```python
from build123d import *

# Parameters (mm, degrees)
SKETCH1_R           = 1.6
BOSS_EXTRUDE1_DEPTH = 5
SKETCH2_R           = 2.5
CUT_EXTRUDE1_DEPTH  = 17.770509831


with BuildPart() as part:
    # Sketch1 → Boss-Extrude1 (new body)
    with BuildSketch(Plane(origin=(0, 0, 0), x_dir=(1, 0, 0), z_dir=(0, 1, 0))):
        with BuildLine():
            Line((-7.5, 5), (7.5, 5))
            ThreePointArc((7.5, 5), (12.5, 0), (7.5, -5))
            Line((7.5, -5), (-7.5, -5))
            ThreePointArc((-7.5, -5), (-12.5, 0), (-7.5, 5))
        make_face()
        with Locations(Location((-7.5, 0, 0), (0, 0, 270))):
            Circle(SKETCH1_R, mode=Mode.SUBTRACT)
        with Locations(Location((7.5, 0, 0), (0, 0, 270))):
            Circle(SKETCH1_R, mode=Mode.SUBTRACT)
    extrude(amount=BOSS_EXTRUDE1_DEPTH)

    # Sketch2 → Cut-Extrude1 (cut, through all)
    with BuildSketch(Plane.XY.offset(5)):
        with Locations((0, -1)):
            Circle(SKETCH2_R)
    extrude(amount=-CUT_EXTRUDE1_DEPTH, mode=Mode.SUBTRACT)


solid = part.part
```
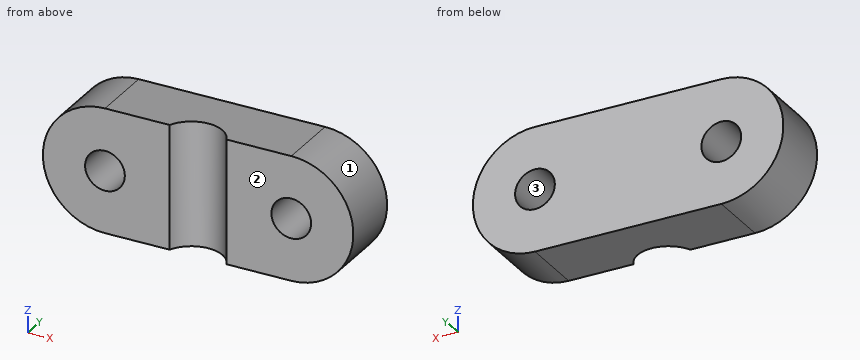
Geometry: final body of the model. Coordinates: model frame, mm. Face numbers are marked on the shaded views. Round coordinates to 2 decimals unless told otherwise and drop trailing zeros. Order: outer loops, then holes, each group sorted by start corner. A loop starts at its lowest first (then second) coordinate and runs counter-clockwise, first axis right, second up. Notation, with made-up numbers: (44.5, 25) -> (92.5, 25) arc R23 ccw to (92.5, 60) -> close; hole circle Ø11 at (-29.5, 41). An arc over 180 degrees is marked (long way). Use CSV: the item, a comma, the result in double quotes. Start each with the question number.
1) Section D-D (y = 3.95). Return the cut outline in (x, z).
2) Section C-C (x = -6.25). Return the cut outline in (y, z), and give its area (3 significant figures).
3) Section A-A (y = 0.8). Return the cut outline in (x, z).
4) Draft query along X for the marked faces 1, 2 and 3. Return one class per face: +X half, -X half, draft (parallel to the pull), parting line (faces both ways), or undercut.
5) Material intervals for line 1 along X through (y, z) = (3.6, 0); line 2 along X through (y, z) = (2.9, -1.25); line 3 along X through (y, z) = (1.2, 0), sorted ascending. Write a range as from..to.
6) Section B-B (z = 0). Return the cut outline in (x, y).
Returned:
1,outline,"(-7.5, -5) -> (7.5, -5) arc R5 ccw to (7.5, 5) -> (-7.5, 5) arc R5 ccw to start; hole circle Ø3.2 at (-7.5, 0); hole circle Ø3.2 at (7.5, 0)"
2,outline,"(0, -5) -> (5, -5) -> (5, -1) -> (0, -1) -> close; (0, 1) -> (5, 1) -> (5, 5) -> (0, 5) -> close"
2,area,"40.0 mm²"
3,outline,"(-7.5, -5) -> (-1.73, -5) -> (-1.73, 5) -> (-7.5, 5) arc R5 ccw to start; (1.73, -5) -> (7.5, -5) arc R5 ccw to (7.5, 5) -> (1.73, 5) -> close; hole circle Ø3.2 at (-7.5, 0); hole circle Ø3.2 at (7.5, 0)"
4,face 1,"+X half"
4,face 2,"draft"
4,face 3,"undercut"
5,line 1,"x = -12.5..-9.1, -5.9..5.9, 9.1..12.5"
5,line 2,"x = -12.34..-8.5, -6.5..6.5, 8.5..12.34"
5,line 3,"x = -12.5..-9.1, -5.9..-1.19, 1.19..5.9, 9.1..12.5"
6,outline,"(-12.5, 0) -> (-9.1, 0) -> (-9.1, 5) -> (-12.5, 5) -> close; (-5.9, 0) -> (-2.29, 0) arc R2.5 cw to (2.29, 0) -> (5.9, 0) -> (5.9, 5) -> (-5.9, 5) -> close; (9.1, 0) -> (12.5, 0) -> (12.5, 5) -> (9.1, 5) -> close"
